Verification items for the finished model (mm, model axes). Coordinates: 2 decimals unless noted, no trailing zeros. Loops run counter-clockwise (first coordinate to the right, second up) from the corner with the lowest first, then second, coordinate; pieces in that order, holes last. Notation, with made-up numbers: (-33.75, -2) - (25.25, -2) arc R21 cw to (25.25, 21) - close; hole circle Ø1 at (37, 41.25). An arc over 180 degrees is marked (long way). One line per item, written item: value. Start each with the question number.
(1) Section check A-A (x = 0). Record the boundary of the cut face in (y, z).
(2) Thickness scan on probe 1 along Y at (x, z) = (0, 1.5); probe 2 along Y at (x, z) = (1.5, 3.75); probe 3 along X at (y, z) = (-13, 1.25). Record the ranges inside material, lowest first. Write a range as [from, to].
(3) Section check C-C (x = 14.5). Record the boundary of the cut face in (y, z).
(4) Draft check along Y on faces 1 (the face through (23.016, 7.248, 2.166)), 2 (the face through (0, -5, 4.394)), 3 (the face through (-0.867, -3.905, 2.166)). Enter one of: +Y half, -Y half, draft (parallel to the pull), parting line (faces both ways), or undercut.
(5) Section check D-D (z = 0.9). Record the boundary of the cut face in (x, y), plus the area to 3 significant figures.
(6) Section check B-B (y = 0). Record the boundary of the cut face in (x, z).
```python
from build123d import *

# Parameters (mm, degrees)
SKETCH1_R           = 24.13
SKETCH1_R_2         = 2.0828
SKETCH1_R_3         = 4
BOSS_EXTRUDE1_DEPTH = 4.3942


with BuildPart() as part:
    # Sketch1 → Boss-Extrude1 (new body)
    with BuildSketch(Plane.XY):
        Circle(SKETCH1_R)
        with Locations((0, 15.24)):
            Circle(SKETCH1_R_2, mode=Mode.SUBTRACT)
        with Locations((14.494101308, 4.709418994)):
            Circle(SKETCH1_R_2, mode=Mode.SUBTRACT)
        with Locations((8.957847245, -12.329418994)):
            Circle(SKETCH1_R_2, mode=Mode.SUBTRACT)
        with Locations((-8.957847245, -12.329418994)):
            Circle(SKETCH1_R_2, mode=Mode.SUBTRACT)
        with Locations((-14.494101308, 4.709418994)):
            Circle(SKETCH1_R_2, mode=Mode.SUBTRACT)
        Circle(SKETCH1_R_3, mode=Mode.SUBTRACT)
    extrude(amount=BOSS_EXTRUDE1_DEPTH)


solid = part.part
```
Responses:
1. outline: (-24.13, 0) - (-4, 0) - (-4, 4.39) - (-24.13, 4.39) - close; (4, 0) - (13.16, 0) - (13.16, 4.39) - (4, 4.39) - close; (17.32, 0) - (24.13, 0) - (24.13, 4.39) - (17.32, 4.39) - close
2. probe 1: y = [-24.13, -4], [4, 13.16], [17.32, 24.13]
2. probe 2: y = [-24.08, -3.71], [3.71, 13.79], [16.69, 24.08]
2. probe 3: x = [-20.33, -10.93], [-6.99, 6.99], [10.93, 20.33]
3. outline: (-19.29, 0) - (2.63, 0) - (2.63, 4.39) - (-19.29, 4.39) - close; (6.79, 0) - (19.29, 0) - (19.29, 4.39) - (6.79, 4.39) - close
4. face 1: parting line
4. face 2: draft
4. face 3: undercut
5. outline: circle Ø48.26 at (0, 0); hole circle Ø4.17 at (-14.49, 4.71); hole circle Ø4.17 at (-8.96, -12.33); hole circle Ø8 at (0, 0); hole circle Ø4.17 at (0, 15.24); hole circle Ø4.17 at (8.96, -12.33); hole circle Ø4.17 at (14.49, 4.71)
5. area: 1,710 mm²
6. outline: (-24.13, 0) - (-4, 0) - (-4, 4.39) - (-24.13, 4.39) - close; (4, 0) - (24.13, 0) - (24.13, 4.39) - (4, 4.39) - close
